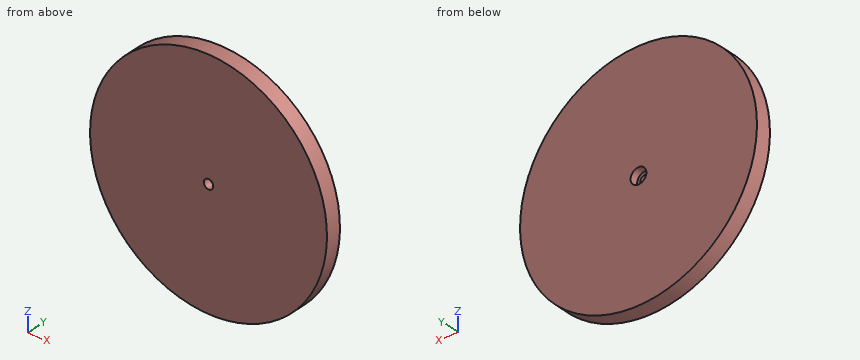
from build123d import *

# Parameters (mm, degrees)
SKETCH_1_R          = 15
EXTRUDE_1_DEPTH     = 2
SKETCH_2_R          = 0.6
CUT_EXTRUDE_1_DEPTH = 22.307275753
SKETCH_2_3_R        = 1
CUT_EXTRUDE_2_DEPTH = 1


with BuildPart() as part:
    # Sketch 1 → Extrude 1 (new body)
    with BuildSketch(Plane(origin=(0, 0, 0), x_dir=(1, 0, 0), z_dir=(0, 1, 0))):
        with Locations(Location((0, 0, 0), (0, 0, 270))):
            Circle(SKETCH_1_R)
    extrude(amount=EXTRUDE_1_DEPTH)

    # Sketch 2 → Cut-Extrude 1 (cut, through all)
    with BuildSketch(Plane(origin=(0, 2, 0), x_dir=(1, 0, 0), z_dir=(0, 1, 0))):
        with Locations(Location((0, 0, 0), (0, 0, 270))):
            Circle(SKETCH_2_R)
    extrude(amount=-CUT_EXTRUDE_1_DEPTH, mode=Mode.SUBTRACT)

    # Sketch 2_3 → Cut-Extrude 2 (cut)
    with BuildSketch(Plane(origin=(0, 2, 0), x_dir=(1, 0, 0), z_dir=(0, 1, 0))):
        with Locations(Location((0, 0, 0), (0, 0, 270))):
            Circle(SKETCH_2_3_R)
    extrude(amount=-CUT_EXTRUDE_2_DEPTH, mode=Mode.SUBTRACT)


solid = part.part
The model under review builds one solid part; all positions refer to its coordinate system, in mm. Coordinates: 2 decimals unless noted, no trailing zeros. Write each loop counter-clockwise with the first axis right and the second up, starting at its lowest first coordinate (ties: lowest second). Pieces come first, ordered by that corner, then holes. Notation, with made-up numbers: (-16, -12.5) - (-5, -12.5) arc R25 ccw to (-5, 22.5) - close; hole circle Ø6 at (84.25, -40). An arc over 180 degrees is marked (long way). Answer as CSV lines item,"result".
(1) We need section C-C (y = 0.45). Give the boundary of the cut face in (x, z), plus the area to 3 significant figures.
Data:
outline,"circle Ø30 at (0, 0); hole circle Ø1.2 at (0, 0)"
area,"706 mm2"
(2) Clearance check with flat-ended pins moving along their axes: pin 1 Ø1 at (y, z) = (1.5, 3.5) entering from -X; pin 2 Ø1 at (y, z) = (1, -11.5) entering from +X. State where each tip first meets the part, or that it passes through.
Data:
pin 1,"stops at x = -14.7"
pin 2,"stops at x = 10.2"
(3) We need section D-D (z = 12). Give the boundary of the cut face in (x, y).
Data:
outline,"(-9, 0) - (9, 0) - (9, 2) - (-9, 2) - close"
(4) We need section A-A (x = 0). Give the boundary of the cut face in (y, z), plus the area to 3 significant figures.
Data:
outline,"(0, -15) - (2, -15) - (2, -1) - (1, -1) - (1, -0.6) - (0, -0.6) - close; (0, 0.6) - (1, 0.6) - (1, 1) - (2, 1) - (2, 15) - (0, 15) - close"
area,"56.8 mm2"
(5) We need section B-B (z = 0). Give the boundary of the cut face in (x, y).
Data:
outline,"(-15, 0) - (-0.6, 0) - (-0.6, 1) - (-1, 1) - (-1, 2) - (-15, 2) - close; (0.6, 0) - (15, 0) - (15, 2) - (1, 2) - (1, 1) - (0.6, 1) - close"
(6) For line 1 along X through (y, z) = (0.3, 0); line 2 along X through (y, z) = (1.7, 0); line 3 along Z through (x, y) = (13, 1.8), list the stretches that pass through material, from the lowest coordinate up. Write a range as [from, to].
Data:
line 1,"x = [-15, -0.6], [0.6, 15]"
line 2,"x = [-15, -1], [1, 15]"
line 3,"z = [-7.48, 7.48]"
